The figure shows three views and two pictorial views of one solid part (mm, origin at its lowest corner). Answer the questions. Give positions to 0.01 mm unless a question says otherwise; leave off trailing zeros. Order: outer loops, then holes, each group sorted by start corner. A loop starts at its lowest first (then second) coordinate and runs counter-clockwise, first axis right, second up. Notation, with made-up numbers: (-40, 63.25) - (2, 63.25) arc R15 cw to (2, 88.25) - close; hole circle Ø8 at (-19, 37.5). An arc over 180 degrees is marked (long way). Use a Markdown table: item, result. Add a question column.
1. A cutting plane is placed at C-C on z = 45.5. Determine the outline of the cut face in (x, y).
2. Consider L1, parallel to Z at x = 87.5, y = 2.45; L2, parallel to X at y = 1.45, z = 149. Determine where each line is inside the solid, lowest interval first.
3. A cutting plane is placed at D-D on z = 233.5. Determine the outline of the cut face in (x, y).
4. A cutting plane is placed at B-B on y = 2.1. State how many separate pieces and enclosed holes the cut face has, and give its area (3 significant figures).
5. A cutting plane is placed at A-A on z = 150. Determine the outline of the cut face in (x, y).
6. Flat-ended cylindrical pins translate along their axes: P1, Ø1.5, axis at x = 79, y = 2, coming from the -Z side; P2, Ø20, axis at x = 150, z = 150, coming from the +Y side; P3, Ø1.5, axis at y = 1.5, z = 115.5, coming from the +X side. Find the tip coordinate at first contact, or state that the pin passes through.
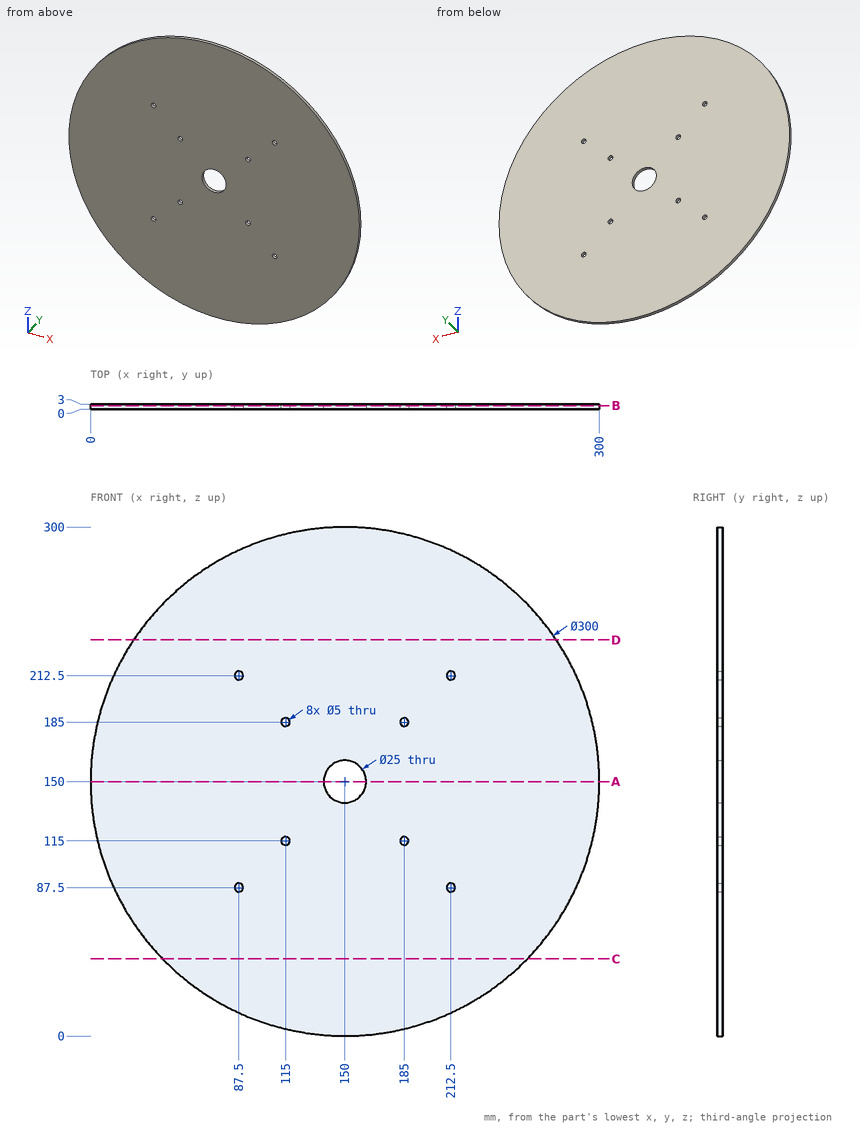
Output values:
| question | item | result |
|---|---|---|
| 1 | outline | (42.39, 0) - (257.61, 0) - (257.61, 3) - (42.39, 3) - close |
| 2 | L1 | 13.64 to 85, 90 to 210, 215 to 286.36 |
| 2 | L2 | 0 to 137.54, 162.46 to 300 |
| 3 | outline | (25.39, 0) - (274.61, 0) - (274.61, 3) - (25.39, 3) - close |
| 4 | separate pieces | 1 |
| 4 | enclosed holes | 9 |
| 4 | area | 70,000 mm² |
| 5 | outline | (0, 0) - (137.5, 0) - (137.5, 3) - (0, 3) - close; (162.5, 0) - (300, 0) - (300, 3) - (162.5, 3) - close |
| 6 | P1 | z = 17.47 |
| 6 | P2 | through |
| 6 | P3 | x = 296.15 |
